Build history of the part. All positions in model axes, mm. A direction names the side the tool comes from. Coordinates: 2 decimals unless noted, no trailing zeros. Write each loop counter-clockwise with the first axis right and the second up, starting at its lowest first coordinate (ties: lowest second). Pieces come first, ordered by that corner, then holes. Notation, with made-up numbers: (42.25, 58) -> (86.25, 58) arc R20 cw to (86.25, 81) -> close; hole circle Ø8 at (49, 12). An arc over 180 degrees is marked (long way). Write each question's results on one line, items separated by ' | '. Start each with the question number.
Q1. Saw through at A-A on z = 35. Give the cut face in (x, y).
Q2. Saw through at C-C on x = 29. Give the cut face in (y, z), and give its area (3 significant figures).
Q3. Saw through at D-D on y = -28.5. Give the cut face in (x, z), and give its area (3 significant figures).
Q4. Tool access for faces 1 (the face through (-26.549, -22.528, 8.884)), 2 (the face through (-17.5, -13, 22)), 3 (the face through (2, -17, 45)): list every direction of +Z, -Z, +X, -X, +Y, -Y with a clear straight run to the whole face (end or side of a thin tool).
Q5. Two-plate mould, pull along Y, no slides. Class faces 4 (the face through (-26.549, -12.472, 36.116)), 5 (the face through (24.475, -25.019, 22.185)), 6 (the face through (2, -16, 4)): released by +Y, released by -Y, zero draft, split by the parting line, or undercut.
Q6. Drill centre lines: line 1 (Z direction, x = 20, y = -2); line 2 (Y direction, x = -28.5, z = 10); line 3 (X direction, y = -18.5, z = 10). Where is each one in solid material? Low to high.
Q7. Saw through at B-B on y = -9. Give the cut face in (x, z).
Q8. Drop flat-ended pins along their axis: pin 1 Ø6 at (y, z) = (-17.5, 35) entering from -X; pin 2 Ø1.5 at (x, z) = (14.5, 14) entering from +Y; pin 3 Ø10 at (y, z) = (-30, 24) entering from +X. Give the stop position or say it passes through.
from build123d import *

# Parameters (mm, degrees)
BOSS_EXTRUDE1_DEPTH = 45
SKETCH2_W           = 31
SKETCH2_H           = 37
BOSS_EXTRUDE3_START = -45
BOSS_EXTRUDE3_DEPTH = 45
SKETCH4_R           = 5.15
CUT_EXTRUDE1_DEPTH  = 12
SKETCH5_W           = 5
SKETCH5_H           = 35
CUT_EXTRUDE2_DEPTH  = 67.895440801


with BuildPart() as part:
    # Sketch1 → Boss-Extrude1 (new body)
    with BuildSketch(Plane.XY):
        with BuildLine():
            Line((35, 0), (-35, 0))
            ThreePointArc((-35, 0), (0, -35), (35, 0))
        make_face()
    extrude(amount=BOSS_EXTRUDE1_DEPTH)

    # Sketch2 → Cut-Revolve1 (revolve, cut)
    with BuildSketch(Plane(origin=(0, 0, 0), x_dir=(1, 0, 0), z_dir=(0, 1, 0))):
        with Locations((-15.5, -22.5)):
            Rectangle(SKETCH2_W, SKETCH2_H)
    revolve(axis=Axis((0, 0, 0), (0, 0, 1)), mode=Mode.SUBTRACT)

    # Sketch3 → Boss-Extrude3 (add)
    with BuildSketch(Plane.XY.offset(45).offset(BOSS_EXTRUDE3_START)):
        with BuildLine():
            Line((-17.5, -35), (-17.5, -30.310889132))
            ThreePointArc((-17.5, -30.310889132), (-30.310889132, -17.5), (-35, 0))
            Line((-35, 0), (-35, -35))
            Line((-35, -35), (-17.5, -35))
        make_face()
        with BuildLine():
            ThreePointArc((0, -35), (-9.058666579, -33.80740392), (-17.5, -30.310889132))
            Line((-17.5, -30.310889132), (-17.5, -35))
            Line((-17.5, -35), (0, -35))
        make_face()
        with BuildLine():
            Line((-17.5, -30.310889132), (-17.5, 0))
            Line((-17.5, 0), (-35, 0))
            ThreePointArc((-35, 0), (-30.310889132, -17.5), (-17.5, -30.310889132))
        make_face()
    extrude(amount=BOSS_EXTRUDE3_DEPTH)

    # Sketch4 → Cut-Extrude1 (cut)
    with BuildSketch(Plane.ZY.offset(35)):
        with Locations((10, -17.5)):
            Circle(SKETCH4_R)
        with Locations(Location((35, -17.5, 0), (0, 0, 180))):
            Circle(SKETCH4_R)
    extrude(amount=-CUT_EXTRUDE1_DEPTH, mode=Mode.SUBTRACT)

    # Sketch5 → Cut-Extrude2 (cut, through all)
    with BuildSketch(Plane(origin=(0, 0, 0), x_dir=(-1, 0, 0), z_dir=(0, 0, -1))):
        with Locations((32.5, -17.5)):
            Rectangle(SKETCH5_W, SKETCH5_H)
    extrude(amount=-CUT_EXTRUDE2_DEPTH, mode=Mode.SUBTRACT)


solid = part.part
Returned:
1) outline: (-30, -35) -> (0, -35) arc R35 ccw to (35, 0) -> (31, 0) arc R31 cw to (-17.5, -25.59) -> (-17.5, 0) -> (-30, 0) -> (-30, -12.35) -> (-23, -12.35) -> (-23, -22.65) -> (-30, -22.65) -> close
2) outline: (-19.6, 0) -> (0, 0) -> (0, 4) -> (-10.95, 4) -> (-10.95, 41) -> (0, 41) -> (0, 45) -> (-19.6, 45) -> close | area: 477 mm2
3) outline: (-30, 0) -> (20.32, 0) -> (20.32, 45) -> (-30, 45) -> close; hole (-12.2, 4) -> (12.2, 4) -> (12.2, 41) -> (-12.2, 41) -> close | area: 1,360 mm2
4) face 1: -X | face 2: +Y | face 3: +Z, +X, -X, +Y, -Y
5) face 4: undercut | face 5: released by -Y | face 6: zero draft
6) line 1: z = 0 to 4, 41 to 45 | line 2: y = -35 to -22.65, -12.35 to 0 | line 3: x = -23 to -17.5, 24.87 to 29.71
7) outline: (-30, 0) -> (33.82, 0) -> (33.82, 45) -> (-30, 45) -> close; hole (-17.5, 4) -> (29.66, 4) -> (29.66, 41) -> (-17.5, 41) -> close
8) pin 1: stops at x = -23 | pin 2: stops at y = -26.99 | pin 3: stops at x = 24.49
